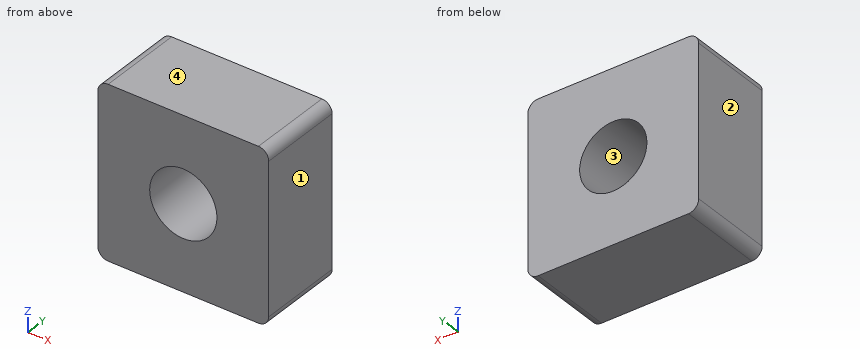
from build123d import *

# Parameters (mm, degrees)
BOSS_EXTRUDE1_DEPTH   = 6.35
M6X1_0_TAPPED_HOLE1_D = 5


with BuildPart() as part:
    # Sketch1 → Boss-Extrude1 (new body)
    with BuildSketch(Plane(origin=(0, 0, 0), x_dir=(1, 0, 0), z_dir=(0, 1, 0))):
        with BuildLine():
            Line((-5.588, -6.35), (5.588, -6.35))
            ThreePointArc((5.588, -6.35), (6.126815367, -6.126815367), (6.35, -5.588))
            Line((6.35, -5.588), (6.35, 5.588))
            ThreePointArc((6.35, 5.588), (6.126815367, 6.126815367), (5.588, 6.35))
            Line((5.588, 6.35), (-5.588, 6.35))
            ThreePointArc((-5.588, 6.35), (-6.126815367, 6.126815367), (-6.35, 5.588))
            Line((-6.35, 5.588), (-6.35, -5.588))
            ThreePointArc((-6.35, -5.588), (-6.126815367, -6.126815367), (-5.588, -6.35))
        make_face()
    extrude(amount=BOSS_EXTRUDE1_DEPTH)

    # M6x1.0 Tapped Hole1 (through all)
    with Locations(Plane(origin=(0, 6.35, 0), x_dir=(1, 0, 0), z_dir=(0, 1, 0))):
        with Locations((0, 0)):
            Hole(M6X1_0_TAPPED_HOLE1_D / 2)


solid = part.part
Part model, mm, in its own coordinate system. Face numbers are marked on the shaded views. Give positions to 0.01 mm unless a question says otherwise; leave off trailing zeros. Loops run counter-clockwise (first coordinate to the right, second up) from the corner with the lowest first, then second, coordinate; pieces in that order, holes last. Notation, with made-up numbers: M 38,43 L 72,43 A19 ccw 72,56 Z; hole C -2,33 d3. An arc over 180 degrees is marked long. Put each result on its own line as item: value. Start each with the question number.
1) Flat gauge pin, fed straight in: pin 1 (3 mm diameter, centred on x = 3.5, z = 3, fed in from -Y). Where does the tip first touch, or does it go through?
2) Saw through at C-C (y = 5.25). List the corners of the cut face in (x, z), then the cut area to 3 significant figures.
3) Probe probe 1 along Z at (x, y) = (0, 3); probe 2 along Z at (x, y) = (2, 2.5); probe 3 along X at (y, z) = (2.75, -1.5). List the from-to ranges inside material, lowest first.
4) Pull direction X, two halves, no side cores. Call the marked faces 1, 2, 3 and 4: +X half, -X half, draft (parallel to the pull), parting line (faces both ways), or undercut.
5) Saw through at A-A (x = 2). List the corners of the cut face in (y, z).
6) Saw through at B-B (z = -2). List the corners of the cut face in (x, y), then the cut area to 3 significant figures.
Numbers:
1. pin 1: y = 0
2. outline: M -6.35,-5.59 A0.76 ccw -5.59,-6.35 L 5.59,-6.35 A0.76 ccw 6.35,-5.59 L 6.35,5.59 A0.76 ccw 5.59,6.35 L -5.59,6.35 A0.76 ccw -6.35,5.59 Z; hole C 0,0 d5
2. area: 141 mm^2
3. probe 1: -6.35 to -2.5, 2.5 to 6.35
3. probe 2: -6.35 to -1.5, 1.5 to 6.35
3. probe 3: -6.35 to -2, 2 to 6.35
4. face 1: +X half
4. face 2: -X half
4. face 3: undercut
4. face 4: draft
5. outline: M 0,-6.35 L 6.35,-6.35 L 6.35,-1.5 L 0,-1.5 Z; M 0,1.5 L 6.35,1.5 L 6.35,6.35 L 0,6.35 Z
6. outline: M -6.35,0 L -1.5,0 L -1.5,6.35 L -6.35,6.35 Z; M 1.5,0 L 6.35,0 L 6.35,6.35 L 1.5,6.35 Z
6. area: 61.6 mm^2
